```python
from build123d import *

# Parameters (mm, degrees)
SKETCH_2_R      = 74.5
SKETCH_2_R_2    = 1.5
SKETCH_2_R_3    = 2.125
SKETCH_2_R_4    = 6
EXTRUDE_1_DEPTH = 3


with BuildPart() as part:
    # 草图2 → 凸台-拉伸1 (new body)
    with BuildSketch(Plane(origin=(0, 0, 0), x_dir=(1, 0, 0), z_dir=(0, 1, 0))):
        with Locations(Location((0, 0, 0), (0, 0, 270))):
            Circle(SKETCH_2_R)
        with Locations(Location((-50.558134855, -50.558134855, 0), (0, 0, 270))):
            Circle(SKETCH_2_R_2, mode=Mode.SUBTRACT)
        with Locations(Location((-71.5, 0, 0), (0, 0, 270))):
            Circle(SKETCH_2_R_2, mode=Mode.SUBTRACT)
        with Locations(Location((0, -71.5, 0), (0, 0, 270))):
            Circle(SKETCH_2_R_2, mode=Mode.SUBTRACT)
        with Locations(Location((50.558134855, -50.558134855, 0), (0, 0, 270))):
            Circle(SKETCH_2_R_2, mode=Mode.SUBTRACT)
        with Locations(Location((-50.558134855, 50.558134855, 0), (0, 0, 270))):
            Circle(SKETCH_2_R_2, mode=Mode.SUBTRACT)
        with Locations(Location((71.5, 0, 0), (0, 0, 270))):
            Circle(SKETCH_2_R_2, mode=Mode.SUBTRACT)
        with Locations(Location((0, 71.5, 0), (0, 0, 270))):
            Circle(SKETCH_2_R_2, mode=Mode.SUBTRACT)
        with Locations(Location((50.558134855, 50.558134855, 0), (0, 0, 270))):
            Circle(SKETCH_2_R_2, mode=Mode.SUBTRACT)
        with Locations(Location((7.75, 6.123393759, 0), (0, 0, 270))):
            Circle(SKETCH_2_R_3, mode=Mode.SUBTRACT)
        with Locations(Location((-7.75, -20.723393759, 0), (0, 0, 270))):
            Circle(SKETCH_2_R_3, mode=Mode.SUBTRACT)
        with Locations(Location((-15.5, -7.3, 0), (0, 0, 270))):
            Circle(SKETCH_2_R_3, mode=Mode.SUBTRACT)
        with Locations(Location((7.75, -20.723393759, 0), (0, 0, 270))):
            Circle(SKETCH_2_R_3, mode=Mode.SUBTRACT)
        with Locations(Location((15.5, -7.3, 0), (0, 0, 270))):
            Circle(SKETCH_2_R_3, mode=Mode.SUBTRACT)
        with Locations(Location((-7.75, 6.123393759, 0), (0, 0, 270))):
            Circle(SKETCH_2_R_3, mode=Mode.SUBTRACT)
        with Locations(Location((0, 0, 0), (0, 0, 270))):
            Circle(SKETCH_2_R_4, mode=Mode.SUBTRACT)
    extrude(amount=EXTRUDE_1_DEPTH)


solid = part.part
```
For this review, take the finished solid that the model builds, in its own axes (mm). Round coordinates to 2 decimals unless told otherwise and drop trailing zeros. Write each loop counter-clockwise with the first axis right and the second up, starting at its lowest first coordinate (ties: lowest second). Pieces come first, ordered by that corner, then holes. Notation, with made-up numbers: (21, 0) -> (66, 0) arc R20 cw to (66, 18) -> close; hole circle Ø11 at (51.5, -35). An arc over 180 degrees is marked (long way). Use one line per item in the form item = value.
Q1. To check wall thickness, follow probe 1 along X at (y, z) = (2, -5.5); probe 2 along Z at (x, y) = (-8.5, 0.3); probe 3 along X at (y, z) = (0.8, 7.3) (3 decimals). State the ranges of each line that lie inside material, in increasing order. Write a range as from..to.
Resolved:
probe_1 = -74.3..-9.78, -5.72..-2.4, 2.4..5.72, 9.78..74.3
probe_2 = -74.01..-8.11, -4.14..18.74, 22.71..74.01
probe_3 = -74.141..-17.625, -13.375..13.375, 17.625..74.141
Q2. The part is to be moulded in two halves that separate along X. For faces 1 (the cylindrical face through (15.593, 1.479, 5.177)), 2 (the cylindrical face through (22.38, 1.48, 71.06)), 3 (the flat face through (-16, 0, -1)), say which applies: released by +X, released by -X, zero draft, split by the parting line, or undercut.
Resolved:
face_1 = undercut
face_2 = split by the parting line
face_3 = zero draft
Q3. Clearance check with flat-ended pins moving along their axes: pin 1 Ø4 at (x, z) = (71.5, 0) entering from -Y; pin 2 Ø1 at (y, z) = (1.5, -13) entering from +X. State where each tip first meets the part, or that it passes through.
Resolved:
pin_1 = 0
pin_2 = 73.44
Q4. Consider section D-D (z = 44.5). State the section outline as (x, y) points.
Resolved:
outline = (-59.75, 0) -> (59.75, 0) -> (59.75, 3) -> (-59.75, 3) -> close
Q5. Consider section A-A (x = 7.75). State the section outline as (y, z) points.
Resolved:
outline = (0, -74.1) -> (3, -74.1) -> (3, -8.25) -> (0, -8.25) -> close; (0, -4) -> (3, -4) -> (3, 18.6) -> (0, 18.6) -> close; (0, 22.85) -> (3, 22.85) -> (3, 74.1) -> (0, 74.1) -> close
Q6. Consider section C-C (x = -44). State the section outline as (y, z) points, then the cut area to 3 significant figures.
Resolved:
outline = (0, -60.12) -> (3, -60.12) -> (3, 60.12) -> (0, 60.12) -> close
area = 361 mm²
Q7. Consider section B-B (y = 1.15). State how many separate pieces and enclosed holes the cut face has, then the cut area to 3 significant figures.
Resolved:
separate_pieces = 1
enclosed_holes = 15
area = 17,200 mm²
